Can you work these out from the model? Positions are in its coordinate system, mm. A direction names the side the tool comes from. Give positions to 0.01 mm unless a question says otherwise; leave off trailing zeros. Order: outer loops, then holes, each group sorted by start corner. A loop starts at its lowest first (then second) coordinate and runs counter-clockwise, first axis right, second up.
Item 1: If we mould it in two halves opening along X, with no side actions, what happens to faces 1 (the flat face through (9.525, 8, -6)), 2 (the flat face through (0.1, 6.35, -10.5)), 3 (the cylindrical face through (0.43, -3.22, -3.86))? For each: +X half, -X half, draft (parallel to the pull), parting line (faces both ways), or undercut.
Item 2: If I drill on line 1 along Y through (x, z) = (8.75, -7); line 2 along X through (y, z) = (-0.75, -7.5) (3 decimals); line 3 along Z through (x, y) = (-2.5, 0.5), over which ranges is the centre line in solid material (lowest first)?
Item 3: Which directions (+Z, -Z, +X, -X, +Y, -Y) give clear straight access to the entire face, cutting with the end or side of a thin tool? Please do faces 4 (the flat face through (0, -6.35, -3)), 5 (the flat face through (15.875, -1, -2)), 6 (the flat face through (-9.525, 0, -6)), 7 (the flat face through (2.5, 0, -5.5)), 8 (the flat face through (15.286, -1.68, -9.389)).
Item 4: I want a section at B-B, the plane y = -4. Write out the boundary of the cut face in (x, z) (3 decimals).
Item 5: I'm going to push flat-ended pins straight in: pin 1 Ø6 at (x, z) = (-0.5, -5.5) entering from -Y; pin 2 Ø6.5 at (x, z) = (-0.127, -6.35) entering from +Y; pin 3 Ø3 at (x, y) = (3.5, 8) entering from -Z; pin 4 Ø3 at (y, z) = (-9, -6.5) entering from -X (3 decimals). Where does each tip first touch, or does it pass through?
Item 6: I want a section at A-A, the plane z = -6.35. Write out the boundary of the cut face in (x, y) (3 decimals), then the cut area to 3 significant figures.
Item 7: I want a section at D-D, the plane x = -5.75. Write out the boundary of the cut face in (y, z), then the cut area to 3 significant figures.
Item 8: I want a section at C-C, the plane y = -9.5. Write out the boundary of the cut face in (x, z) (3 decimals), then the cut area to 3 significant figures.
```python
from build123d import *

# Parameters (mm, degrees)
SALIENTE_EXTRUIR1_DEPTH                              = 12.7
REFRENTADO_PARA_TORNILLO_CON_CABEZA_HUEC_D           = 5.1054
REFRENTADO_PARA_TORNILLO_CON_CABEZA_HUEC_CBORE_D     = 7.9375
REFRENTADO_PARA_TORNILLO_CON_CABEZA_HUEC_CBORE_DEPTH = 6.35
REFRENTADO_PARA_TORNILLO_CON_CABEZA_2_D              = 4.2672
REFRENTADO_PARA_TORNILLO_CON_CABEZA_2_CBORE_D        = 5.588
REFRENTADO_PARA_TORNILLO_CON_CABEZA_2_CBORE_DEPTH    = 22.352
CORTAR_EXTRUIR4_DEPTH                                = 22.352
CORTAR_EXTRUIR5_DEPTH                                = 33.139030617
CORTAR_EXTRUIR2_DEPTH                                = 6.35


with BuildPart() as part:
    # Croquis1 → Saliente-Extruir1 (new body)
    with BuildSketch(Plane.XY):
        Polygon((-9.525, 6.35), (-9.525, -6.35), (9.525, -6.35), (9.525, -12.7), (15.875, -12.7), (15.875, 12.192), (9.525, 12.192), (9.525, 6.35), align=None)
    extrude(amount=-SALIENTE_EXTRUIR1_DEPTH)

    # Refrentado para tornillo con cabeza huec (through all)
    with Locations(Plane(origin=(0, 6.35, 0), x_dir=(1, 0, 0), z_dir=(0, 1, 0))):
        with Locations((-0.127, 6.35)):
            CounterBoreHole(REFRENTADO_PARA_TORNILLO_CON_CABEZA_HUEC_D / 2, REFRENTADO_PARA_TORNILLO_CON_CABEZA_HUEC_CBORE_D / 2, REFRENTADO_PARA_TORNILLO_CON_CABEZA_HUEC_CBORE_DEPTH)

    # Refrentado para tornillo con cabeza  2 (through all)
    with Locations(Plane(origin=(0, -12.7, 0), x_dir=(-1, 0, 0), z_dir=(0, -1, 0))):
        with Locations((-16.0528, 6.35)):
            CounterBoreHole(REFRENTADO_PARA_TORNILLO_CON_CABEZA_2_D / 2, REFRENTADO_PARA_TORNILLO_CON_CABEZA_2_CBORE_D / 2, REFRENTADO_PARA_TORNILLO_CON_CABEZA_2_CBORE_DEPTH)

    # Croquis12 → Cortar-Extruir4 (cut)
    with BuildSketch(Plane.XZ.offset(12.7)):
        Polygon((15.875, -9.977962986), (14.6812, -8.784162986), (15.875, -8.784162986), align=None)
        Polygon((15.875, -3.915837014), (15.875, -2.722037014), (14.6812, -3.915837014), align=None)
    extrude(amount=-CORTAR_EXTRUIR4_DEPTH, mode=Mode.SUBTRACT)

    # Croquis13 → Cortar-Extruir5 (cut, through all)
    with BuildSketch(Plane.XZ.offset(12.7)):
        Polygon((15.875, -3.966896317), (15.5702, -4.271696317), (15.875, -4.271696317), align=None)
        Polygon((15.875, -8.428303683), (15.875, -8.733103683), (15.5702, -8.428303683), align=None)
    extrude(amount=-CORTAR_EXTRUIR5_DEPTH, mode=Mode.SUBTRACT)

    # Croquis21 → Cortar-Revolución12 (revolve, cut)
    with BuildSketch(Plane.XY.offset(-6.35)):
        Polygon((13.5382, 12.192), (5.6007, 7.422668836), (5.6007, 12.192), align=None)
    revolve(axis=Axis((15.621, 12.192, -6.35), (0, -1, 0)), mode=Mode.SUBTRACT)

    # Croquis5 → Cortar-Extruir2 (cut)
    with BuildSketch(Plane(origin=(15.875, 0, 0), x_dir=(0, 0, -1), z_dir=(1, 0, 0))):
        Polygon((8.472730115, 12.192), (12.7, 9.652), (12.7, 12.192), align=None)
        Polygon((4.227269885, 12.192), (0, 9.652), (0, 12.192), align=None)
    extrude(amount=-CORTAR_EXTRUIR2_DEPTH, mode=Mode.SUBTRACT)


solid = part.part
```
Results list:
1. face 1: -X half
1. face 2: draft
1. face 3: undercut
2. line 1: y = -6.35 to 6.35
2. line 2: x = -9.525 to -2.406, 2.152 to 13.506
2. line 3: z = -12.7 to -9.53, -3.17 to 0
3. face 4: +Z, -Z, -X, -Y
3. face 5: +Z, -Z, +X, +Y, -Y
3. face 6: +Z, -Z, -X, +Y, -Y
3. face 7: +Y
3. face 8: +X, -Y
4. outline: (-9.525, -12.7) - (15.875, -12.7) - (15.875, -9.978) - (14.681, -8.784) arc R2.794 cw to (14.681, -3.916) - (15.875, -2.722) - (15.875, 0) - (-9.525, 0) - close; hole circle Ø5.105 at (-0.127, -6.35)
5. pin 1: stops at y = -6.35
5. pin 2: stops at y = 0
5. pin 3: passes through
5. pin 4: stops at x = 9.525
6. outline: (-9.525, -6.35) - (-2.68, -6.35) - (-2.68, 0) - (-4.096, 0) - (-4.096, 6.35) - (-9.525, 6.35) - close; (2.426, -6.35) - (9.525, -6.35) - (9.525, -12.7) - (13.259, -12.7) - (13.259, 9.652) - (13.919, 9.652) - (13.919, 12.192) - (13.538, 12.192) - (9.525, 9.781) - (9.525, 6.35) - (3.842, 6.35) - (3.842, 0) - (2.426, 0) - close
6. area: 249 mm2
7. outline: (-6.35, -12.7) - (6.35, -12.7) - (6.35, 0) - (-6.35, 0) - close
7. area: 161 mm2
8. outline: (9.525, -12.7) - (15.875, -12.7) - (15.875, -9.978) - (14.681, -8.784) arc R2.794 cw to (14.681, -3.916) - (15.875, -2.722) - (15.875, 0) - (9.525, 0) - close
8. area: 68.5 mm2
